```python
from build123d import *

# Parameters (mm, degrees)
F0_R        = 95.337967
F0_R_2      = 72.892959
F1_DEPTH    = 254
F1_FACE_R   = 95.337967
F1_FACE_R_2 = 72.892959
F2_DEPTH    = 254
F4_D        = 15.875


with BuildPart() as f1:
    # F0 (on Front) → F1 (new body)
    with BuildSketch(Plane.XZ):
        Circle(F0_R)
        Circle(F0_R_2, mode=Mode.SUBTRACT)
    extrude(amount=F1_DEPTH)

    # F1_face (on face) → F2 (join)
    with BuildSketch(Plane.XZ.offset(254)):
        Circle(F1_FACE_R)
        Circle(F1_FACE_R_2, mode=Mode.SUBTRACT)
    extrude(amount=F2_DEPTH)

    # F4 (through all)
    with Locations(Plane.XZ.offset(508)):
        with Locations((-59.389438, 57.769768), (-84.084906, 0), (0, 83.347216), (56.811582, 61.297689), (83.712012, 0), (63.646935, -54.903328), (0, -85.552171), (-51.010616, -66.369079)):
            Hole(F4_D / 2)


solid = f1.part
```
Read the model definition and answer for the solid it produces. Units are mm, in the model's axes. Give positions to 0.01 mm unless a question says otherwise; leave off trailing zeros. Write each loop counter-clockwise with the first axis right and the second up, starting at its lowest first coordinate (ties: lowest second). Pieces come first, ordered by that corner, then holes. Notation, with made-up numbers: (55.5, 6.5) -> (65.5, 6.5) arc R23 ccw to (65.5, 42.5) -> close; hole circle Ø3 at (19, 1.25). An arc over 180 degrees is marked (long way). Answer in a Markdown table with one row per item.
1) Section B-B on z = 0 is taken. Give the vertices of the cut face in (x, y).
Results list:
| item | result |
|---|---|
| outline | (-95.34, -508) -> (-92.02, -508) -> (-92.02, 0) -> (-95.34, 0) -> close; (-76.15, -508) -> (-72.89, -508) -> (-72.89, 0) -> (-76.15, 0) -> close; (72.89, -508) -> (75.77, -508) -> (75.77, 0) -> (72.89, 0) -> close; (91.65, -508) -> (95.34, -508) -> (95.34, 0) -> (91.65, 0) -> close |
2) Section A-A on x = 0 is taken. Give the vertices of the cut face in (y, z), plus the area to 3 significant figures.
Results list:
| item | result |
|---|---|
| outline | (-508, -95.34) -> (0, -95.34) -> (0, -93.49) -> (-508, -93.49) -> close; (-508, -77.61) -> (0, -77.61) -> (0, -72.89) -> (-508, -72.89) -> close; (-508, 72.89) -> (0, 72.89) -> (0, 75.41) -> (-508, 75.41) -> close; (-508, 91.28) -> (0, 91.28) -> (0, 95.34) -> (-508, 95.34) -> close |
| area | 6,680 mm^2 |
3) Straight lines are drawn through the part: line 1 (Z direction, x = 0, y = -251.5); line 2 (X direction, y = -422.5, z = -67); line 3 (X direction, y = -396, z = 51). For each, find the intervals that lie inside material, in ascending order. Write a range as [from, to].
Results list:
| item | result |
|---|---|
| line 1 | [-95.34, -93.49], [-77.61, -72.89], [72.89, 75.41], [91.28, 95.34] |
| line 2 | [-67.83, -58.92], [-43.1, -28.71], [28.71, 67.83] |
| line 3 | [-80.55, -63.53], [-55.25, -52.08], [52.08, 80.55] |
4) Each of these flat-tipped pins is pushed along its axis until it touches: pin 1 Ø9.5 at (x, z) = (0, 83.35) entering from -Y; pin 2 Ø3 at (y, z) = (-171.5, 53) entering from -X; pin 3 Ø8 at (y, z) = (-301, -39) entering from -X; pin 4 Ø12 at (x, y) = (-23.5, -341) entering from -Z. Where does it stop, or does it pass through?
Results list:
| item | result |
|---|---|
| pin 1 | through |
| pin 2 | x = -80.23 |
| pin 3 | x = -88.68 |
| pin 4 | z = -93.72 |
5) Determine the mould class of faces 1 (the cylindrical face through (59.38, -250.44, -48.21)), 2 (the flat face through (-36, 0, 64)), 3 (the cylindrical face through (-20.67, -250.44, -93.07)), 4 (the cylindrical face through (1.72, -250.44, 75.6)) for opening direction Z: released by +Z, released by -Z, zero draft, split by the parting line, or undercut.
Results list:
| item | result |
|---|---|
| face 1 | undercut |
| face 2 | zero draft |
| face 3 | split by the parting line |
| face 4 | undercut |
6) Section C-C on y = -140 is taken. Count the separate pieces of the cut face and the enclosed holes in it, plus the area to 3 significant figures.
Results list:
| item | result |
|---|---|
| separate pieces | 1 |
| enclosed holes | 9 |
| area | 10,300 mm^2 |
7) Section D-D on z = 31 is taken. Give the vertices of the cut face in (x, y).
Results list:
| item | result |
|---|---|
| outline | (-90.16, -508) -> (-65.97, -508) -> (-65.97, 0) -> (-90.16, 0) -> close; (65.97, -508) -> (90.16, -508) -> (90.16, 0) -> (65.97, 0) -> close |
